Verification items for the finished model (mm, model axes). A direction names the side the tool comes from. Give positions to 0.01 mm unless a question says otherwise; leave off trailing zeros. Loops run counter-clockwise (first coordinate to the right, second up) from the corner with the lowest first, then second, coordinate; pieces in that order, holes last. Notation, with made-up numbers: (41.5, -29) - (55.5, -29) arc R3 ccw to (55.5, -25) - close; hole circle Ø5 at (72.25, 71.5). An arc over 180 degrees is marked (long way). One line per question, with ' | ' between items. Start each with the question number.
1. Depth check by flat-ended pin: pin 1 Ø2 at (x, y) = (-5, 58) entering from -Z; pin 2 Ø12 at (x, y) = (18, 16) entering from +Z; pin 3 Ø6 at (y, z) = (26, 3.5) entering from +X; pin 4 Ø2 at (x, z) = (17, 2) entering from +Y. Enter the tip coordinate at first touch or a pass-through.
2. Thickness scan on line 1 along X through (y, z) = (2.25, -18.75); line 2 along Z through (x, y) = (18.75, 1.1); line 3 along Z through (x, y) = (-3.75, 1.2). Record the ranges inside material, lowest first. Write a range as from..to.
3. Section check D-D, the plane x = 18.75. Enter the section's corners in (y, z).
4. Section check C-C, the plane y = 11.5. Enter the section's corners in (x, z), then the cut area to 3 significant figures.
5. Section check B-B, the plane z = 3.75. Enter the section's corners in (x, y), then the cut area to 3 significant figures.
6. Section check A-A, the plane x = -3.75. Enter the section's corners in (y, z).
7. Mould release check, pull along X, two halves, no side actions. Record for faces 5 (the face through (15, 44, 4)), 6 (the face through (-3.945, 1.972, -20.237)), 7 (the face through (-4, 2, -22.5)): +X half, -X half, draft (parallel to the pull), parting line (faces both ways), or undercut.
8. Tool access check on faces 1 (the face through (-4, 44, -15)), 2 (the face through (-7.5, 42, -4)), 3 (the face through (9, 42, 0)), 4 (the face through (20.5, 4, 3.7)). Record the directions out of +Z, -Z, +X, -X, +Y, -Y that give a thin tool (end or side, any length) a straight path to the whole face; none if there is none.
from build123d import *

# Parameters (mm, degrees)
SKETCH1_R           = 1.5
BOSS_EXTRUDE1_DEPTH = 4
BOSS_EXTRUDE2_DEPTH = 82


with BuildPart() as part:
    # Sketch1 → Boss-Extrude1 (new body)
    with BuildSketch(Plane(origin=(0, 0, 0), x_dir=(1, 0, 0), z_dir=(0, 1, 0))):
        Polygon((0, 0), (15, 0), (22.5, 0), (22.5, -7.5), (15, -7.5), (-7.5, -7.5), (-7.5, 22.5), (0, 22.5), (0, 15), align=None)
        with Locations((-3.75, 18.75)):
            Circle(SKETCH1_R, mode=Mode.SUBTRACT)
        with Locations((18.75, -3.75)):
            Circle(SKETCH1_R, mode=Mode.SUBTRACT)
    extrude(amount=BOSS_EXTRUDE1_DEPTH)

    # Sketch3 → Boss-Extrude2 (add)
    with BuildSketch(Plane(origin=(0, 4, 0), x_dir=(1, 0, 0), z_dir=(0, 1, 0))):
        Polygon((0, 0), (0, 15), (-7.5, 15), (-7.5, -7.5), (15, -7.5), (15, 0), align=None)
    extrude(amount=BOSS_EXTRUDE2_DEPTH)


solid = part.part
Results list:
1) pin 1: z = -15 | pin 2: z = 7.5 | pin 3: x = 15 | pin 4: y = 4
2) line 1: -7.5..-5.25, -2.25..0 | line 2: 0..2.25, 5.25..7.5 | line 3: -22.5..-20.25, -17.25..7.5
3) outline: (0, 0) - (4, 0) - (4, 2.25) - (0, 2.25) - close; (0, 5.25) - (4, 5.25) - (4, 7.5) - (0, 7.5) - close
4) outline: (-7.5, -15) - (0, -15) - (0, 0) - (15, 0) - (15, 7.5) - (-7.5, 7.5) - close | area: 281 mm²
5) outline: (-7.5, 0) - (17.25, 0) - (17.25, 4) - (15, 4) - (15, 86) - (-7.5, 86) - close; (20.25, 0) - (22.5, 0) - (22.5, 4) - (20.25, 4) - close | area: 1,950 mm²
6) outline: (0, -22.5) - (4, -22.5) - (4, -20.25) - (0, -20.25) - close; (0, -17.25) - (4, -17.25) - (4, -15) - (86, -15) - (86, 7.5) - (0, 7.5) - close
7) face 5: +X half | face 6: undercut | face 7: draft
8) face 1: -Z, +X, -X, +Y | face 2: +Z, -Z, -X, +Y, -Y | face 3: -Z, +X, +Y, -Y | face 4: +Z, -Z, +X, +Y
